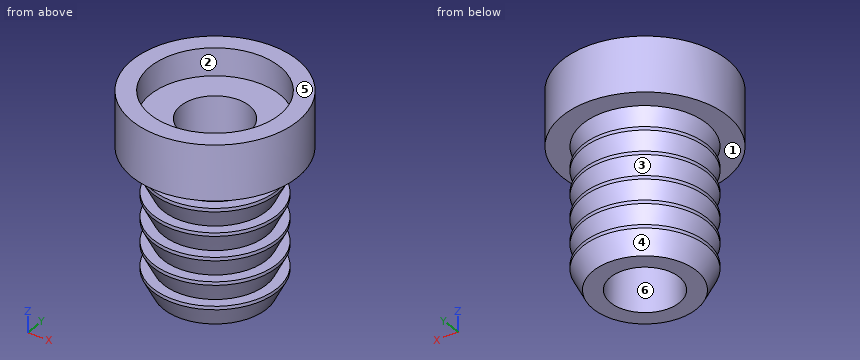
```python
from build123d import *

# Parameters (mm, degrees)
F0_R      = 9
F0_R_2    = 5
F1_DEPTH  = 25
F17_DEPTH = 0.5
F18_R     = 12
F18_R_2   = 9
F19_DEPTH = 4
F20_R     = 9.4
F20_R_2   = 9
F21_DEPTH = 4


with BuildPart() as f1:
    # F0 (on Top) → F1 (new body)
    with BuildSketch(Plane.XY):
        Circle(F0_R)
        Circle(F0_R_2, mode=Mode.SUBTRACT)
    extrude(amount=F1_DEPTH)

    # F15 (on Front) → F16 (revolve, cut)
    with BuildSketch(Plane.XZ):
        Polygon((9, 18), (9, 21), (7.5, 18), align=None)
        Polygon((7.5, 14.5), (9, 14.5), (9, 17.5), align=None)
        Polygon((7.5, 11), (9, 11), (9, 14), align=None)
        Polygon((7.5, 7.5), (9, 7.5), (9, 10.5), align=None)
        Polygon((7.5, 4), (9, 4), (9, 7), align=None)
        Polygon((7.5, 0.5), (9, 0.5), (9, 3.5), align=None)
    revolve(axis=Axis((0, 0, 25), (0, 0, 1)), mode=Mode.SUBTRACT)

    # F17 (cut): a face of the model
    f17_faces = [f1.faces().sort_by_distance(p)[0] for p in [
        (-8.7454415588, 0, 0),
    ]]
    extrude(f17_faces, amount=-F17_DEPTH, mode=Mode.SUBTRACT)

    # F18 (on face) → F19 (join, symmetric)
    with BuildSketch(Plane.XY.offset(25)):
        Circle(F18_R)
        Circle(F18_R_2, mode=Mode.SUBTRACT)
    extrude(amount=F19_DEPTH, both=True)

    # F20 (on face) → F21 (cut, through all)
    with BuildSketch(Plane.XY.offset(29)):
        Circle(F20_R)
        Circle(F20_R_2, mode=Mode.SUBTRACT)
    extrude(amount=-F21_DEPTH, mode=Mode.SUBTRACT)


solid = f1.part
```
Geometry check sheet. Reference: the model listing, model coordinates, mm. Face numbers are marked on the shaded views. A direction names the side the tool comes from. Round coordinates to 2 decimals unless told otherwise and drop trailing zeros. Loops run counter-clockwise (first coordinate to the right, second up) from the corner with the lowest first, then second, coordinate; pieces in that order, holes last. Notation, with made-up numbers: (10, 39.25) - (56, 39.25) arc R26 ccw to (56, 78.25) - close; hole circle Ø11 at (86, 28.5). An arc over 180 degrees is marked (long way). Write each question's results on one line, items separated by ' | '. Start each with the question number.
Q1. Cross-section at C-C on z = 19.5. Enter the section's corners in (x, y).
Q2. Access from +Z, -Z, +X, -X, +Y, -Y to the whole of each face (thin tool, end or side, straight path). Record for the marked faces 1, 2 and 3.
Q3. Thickness scan on line 1 (Y direction, x = 0, z = 27.2); line 2 (Z direction, x = -2.5, y = 8.5); line 3 (Z direction, x = 1.5, y = 10.5). Record the ranges inside material, lowest first. Write a range as [from, to].
Q4. Cross-section at A-A on z = 25.5. Enter the section's corners in (x, y), and give its area (3 significant figures).
Q5. Cross-section at B-B on x = 8.5. State how many separate pieces and enclosed holes the cut face has, and give its area (3 significant figures).
Q6. Gauge pin test, flat ends, axial feed: P1, Ø1, axis at x = -5.5, y = 6.5, coming from the +Z side; P2, Ø7, axis at x = 3, y = 1, coming from the -Z side; P3, Ø1.5, axis at y = 1.5, z = 14, coming from the -X side; P4, Ø3, axis at x = -3, z = 5, coming from the -Y side. Record the tip position at first contact, or that the pin passes through.
Q7. Release check for a two-part mould opening along Y. For the marked faces 4, 5 and 6 record: +Y half, -Y half, draft (parallel to the pull), parting line (faces both ways), or undercut.
Answers below:
1) outline: circle Ø16.5 at (0, 0); hole circle Ø10 at (0, 0)
2) face 1: -Z | face 2: +Z | face 3: none
3) line 1: y = [-12, -9.4], [9.4, 12] | line 2: z = [3.22, 4], [6.72, 7.5], [10.22, 11], [13.72, 14.5], [17.22, 18], [20.72, 25] | line 3: z = [21, 29]
4) outline: circle Ø24 at (0, 0); hole circle Ø18.8 at (0, 0) | area: 175 mm²
5) separate pieces: 6 | enclosed holes: 0 | area: 142 mm²
6) P1: stops at z = 25 | P2: stops at z = 0.5 | P3: stops at x = -8.97 | P4: stops at y = -8.8
7) face 4: parting line | face 5: draft | face 6: undercut
